```python
from build123d import *

# Parameters (mm, degrees)
CROQUIS1_R                      = 14
CROQUIS1_R_2                    = 4
SALIENTE_EXTRUIR1_DEPTH         = 18.9
CHAFL_N1_SIZE                   = 1
CORTAR_EXTRUIR1_REACH           = 44.671
REDONDEO1_R                     = 2
MATRIZC1_COUNT                  = 3
REDONDEO1_OF_MATRIZC1_R         = 2
CROQUIS3_R                      = 4
CORTAR_EXTRUIR2_DEPTH           = 29
TALADRO_ROSCADO_M3_5X0_61_D     = 2.9
TALADRO_ROSCADO_M3_5X0_61_DEPTH = 20
TALADRO_ROSCADO_M3_5X0_61_TIP   = 0.871247898
SALIENTE_EXTRUIR2_START         = -3
CROQUIS6_R                      = 18
CROQUIS6_R_2                    = 4
SALIENTE_EXTRUIR2_DEPTH         = 3
CHAFL_N2_SIZE                   = 0.5
REDONDEO2_R                     = 1


with BuildPart() as part:
    # Croquis1 → Saliente-Extruir1 (new, symmetric)
    with BuildSketch(Plane(origin=(0, 0, 0), x_dir=(0, 1, 0), z_dir=(0, 0, 1))):
        with Locations(Location((0, 0, 0), (0, 0, 270))):
            Circle(CROQUIS1_R)
        with Locations(Location((0, 0, 0), (0, 0, 270))):
            Circle(CROQUIS1_R_2, mode=Mode.SUBTRACT)
    extrude(amount=SALIENTE_EXTRUIR1_DEPTH, both=True)

    # Chaflán1
    chafl_n1_edges = [part.edges().sort_by_distance(p)[0] for p in [
        (-14, 0, 18.9),
    ]]
    chamfer(chafl_n1_edges, length=CHAFL_N1_SIZE)

    # Croquis2 → Cortar-Extruir1 (cut, up to next)
    with BuildSketch(Plane.XY.offset(18.9), mode=Mode.PRIVATE) as cortar_extruir1_sk1:
        with BuildLine():
            Line((4.022667121, 3.750753155), (4.08375287, 10.750486617))
            ThreePointArc((4.08375287, 10.750486617), (0, 11.5), (-4.08375287, 10.750486617))
            Line((-4.08375287, 10.750486617), (-4.022667121, 3.750753155))
            ThreePointArc((-4.022667121, 3.750753155), (0, 5.5), (4.022667121, 3.750753155))
        make_face()
    cortar_extruir1_tool1 = extrude(cortar_extruir1_sk1.sketch, amount=-CORTAR_EXTRUIR1_REACH, mode=Mode.PRIVATE) & part.part
    cortar_extruir1 = cortar_extruir1_tool1.solids().sort_by_distance((0, 8.096632, 18.9))[0]
    add(cortar_extruir1, mode=Mode.SUBTRACT)

    # Redondeo1
    redondeo1_edges = [part.edges().sort_by_distance(p)[0] for p in [
        (4.022667121, 3.750753155, 0),
        (-4.022667121, 3.750753155, 0),
        (-4.08375287, 10.750486617, 0),
        (4.08375287, 10.750486617, 0),
    ]]
    fillet(redondeo1_edges, radius=REDONDEO1_R)

    # MatrizC1: Cortar-Extruir1 ×3 about axis
    matrizc1_axis = Axis((0, 0, 0), (0, 0, 1))
    for i in range(1, MATRIZC1_COUNT):
        add(cortar_extruir1.rotate(matrizc1_axis, i * 360 / MATRIZC1_COUNT), mode=Mode.SUBTRACT)

    # Redondeo1 of MatrizC1
    redondeo1_of_matrizc1_edges = [part.edges().sort_by_distance(p)[0] for p in [
        (-5.259581076, 1.60835534, 0),
        (-1.236913955, -5.359108496, 0),
        (-7.268318079, -8.911877036, 0),
        (-11.352070948, -1.838609581, 0),
        (1.236913955, -5.359108496, 0),
        (5.259581076, 1.60835534, 0),
        (11.352070948, -1.838609581, 0),
        (7.268318079, -8.911877036, 0),
    ]]
    fillet(redondeo1_of_matrizc1_edges, radius=REDONDEO1_OF_MATRIZC1_R)

    # Croquis3 → Cortar-Extruir2 (cut)
    with BuildSketch(Plane(origin=(0, 0, 0), x_dir=(-1, 0, 0), z_dir=(0, 1, 0))):
        with Locations(Location((0, -0.4, 0), (0, 0, 90))):
            Circle(CROQUIS3_R)
    extrude(amount=-CORTAR_EXTRUIR2_DEPTH, mode=Mode.SUBTRACT)

    # Taladro roscado M3.5x0.61
    with Locations(Plane.XY.offset(18.9)):
        with Locations((0, 0), (-9.526279442, 5.5), (9.526279442, 5.5), (0, -11)):
            Hole(TALADRO_ROSCADO_M3_5X0_61_D / 2, depth=TALADRO_ROSCADO_M3_5X0_61_DEPTH)
            with Locations((0, 0, -(TALADRO_ROSCADO_M3_5X0_61_DEPTH + TALADRO_ROSCADO_M3_5X0_61_TIP / 2))):  # 118° drill point
                Cone(0, TALADRO_ROSCADO_M3_5X0_61_D / 2, TALADRO_ROSCADO_M3_5X0_61_TIP, mode=Mode.SUBTRACT)

    # Croquis6 → Saliente-Extruir2 (add)
    with BuildSketch(Plane(origin=(0, 0, -18.9), x_dir=(1, 0, 0), z_dir=(0, 0, -1)).offset(SALIENTE_EXTRUIR2_START)):
        with Locations(Location((0, 0, 0), (0, 0, 180))):
            Circle(CROQUIS6_R)
        Circle(CROQUIS6_R_2, mode=Mode.SUBTRACT)
        with BuildLine():
            Line((-10.049642775, 1.101731175), (-8.258409927, 0.08830039))
            ThreePointArc((-8.258409927, 0.08830039), (-6.485918981, -0.009361739), (-5.333946058, 1.341275307))
            ThreePointArc((-5.333946058, 1.341275307), (-4.763139721, 2.75), (-3.828551518, 3.948695135))
            ThreePointArc((-3.828551518, 3.948695135), (-3.234851986, 5.621651474), (-4.205675344, 7.107842597))
            Line((-4.205675344, 7.107842597), (-5.978948573, 8.152380354))
            ThreePointArc((-5.978948573, 8.152380354), (-7.288087529, 8.407385768), (-8.466451677, 7.782621409))
            ThreePointArc((-8.466451677, 7.782621409), (-9.959292144, 5.75), (-10.973173687, 3.440851528))
            ThreePointArc((-10.973173687, 3.440851528), (-10.92505342, 2.107976061), (-10.049642775, 1.101731175))
        make_face(mode=Mode.SUBTRACT)
        with BuildLine():
            Line((5.978948573, 8.152380354), (4.205675344, 7.107842597))
            ThreePointArc((4.205675344, 7.107842597), (3.234851986, 5.621651474), (3.828551518, 3.948695135))
            ThreePointArc((3.828551518, 3.948695135), (4.763139721, 2.75), (5.333946058, 1.341275307))
            ThreePointArc((5.333946058, 1.341275307), (6.485918981, -0.009361739), (8.258409927, 0.08830039))
            Line((8.258409927, 0.08830039), (10.049642775, 1.101731175))
            ThreePointArc((10.049642775, 1.101731175), (10.92505342, 2.107976061), (10.973173687, 3.440851528))
            ThreePointArc((10.973173687, 3.440851528), (9.959292144, 5.75), (8.466451677, 7.782621409))
            ThreePointArc((8.466451677, 7.782621409), (7.288087529, 8.407385768), (5.978948573, 8.152380354))
        make_face(mode=Mode.SUBTRACT)
        with BuildLine():
            Line((-4.052734583, -7.196142986), (-4.070694202, -9.254111529))
            ThreePointArc((-4.070694202, -9.254111529), (-3.63696589, -10.51536183), (-2.50672201, -11.223472937))
            ThreePointArc((-2.50672201, -11.223472937), (0, -11.5), (2.50672201, -11.223472937))
            ThreePointArc((2.50672201, -11.223472937), (3.63696589, -10.51536183), (4.070694202, -9.254111529))
            Line((4.070694202, -9.254111529), (4.052734583, -7.196142986))
            ThreePointArc((4.052734583, -7.196142986), (3.251066995, -5.612289735), (1.50539454, -5.289970442))
            ThreePointArc((1.50539454, -5.289970442), (0, -5.5), (-1.50539454, -5.289970442))
            ThreePointArc((-1.50539454, -5.289970442), (-3.251066995, -5.612289735), (-4.052734583, -7.196142986))
        make_face(mode=Mode.SUBTRACT)
    extrude(amount=SALIENTE_EXTRUIR2_DEPTH)

    # Chaflán2
    chafl_n2_edges = [part.edges().sort_by_distance(p)[0] for p in [
        (18, 0, -18.9),
        (18, 0, -15.9),
    ]]
    chamfer(chafl_n2_edges, length=CHAFL_N2_SIZE)

    # Redondeo2
    redondeo2_edges = [part.edges().sort_by_distance(p)[0] for p in [
        (-14, 0, -15.9),
    ]]
    fillet(redondeo2_edges, radius=REDONDEO2_R)


solid = part.part
```
Verification items for the finished model (mm, model axes). A direction names the side the tool comes from. Round coordinates to 2 decimals unless told otherwise and drop trailing zeros. Put each result on its own line as item: value. Start each with the question number.
(1) Depth check by flat-ended pin: pin 1 Ø1 at (x, z) = (4.5, 8.5) entering from -Y; pin 2 Ø3 at (y, z) = (-13, 13) entering from +X; pin 3 Ø12 at (x, z) = (-11.5, 9.5) entering from -Y; pin 4 Ø7 at (x, y) = (0, 0) entering from +Z. Enter the tip coordinate at first touch or a pass-through.
(2) Draft check along X on faces 1 (the face through (-13, 8, -15.9)), 2 (the face through (10.975, 5.564, 8.76)), 3 (the face through (13.267, 12.165, -17.386)). Enter one of: +X half, -X half, draft (parallel to the pull), parting line (faces both ways), or undercut.
(3) Tool access check on faces 4 (the face through (10.932, -2.126, -0.265)), 5 (the face through (-1.82, 13.88, 1.73)). Record the directions out of +Z, -Z, +X, -X, +Y, -Y that give a thin tool (end or side, any length) a straight path to the whole face; none if there is none.
(4) Material ranges on line 1 along Y through (x, z) = (0, 4); line 2 along X through (y, z) = (5, 12); line 3 along Z through (x, y) = (0, -7.5), recorded low to high.
(5) Section check A-A (x = 0). State how many separate pieces and enclosed holes the cut face has, then the cut area to 3 significant figures.
Completed:
1. pin 1: stops at y = -13.42
1. pin 2: stops at x = 7.98
1. pin 3: stops at y = -12.87
1. pin 4: passes through
2. face 1: draft
2. face 2: undercut
2. face 3: parting line
3. face 4: +Z, -Z
3. face 5: +Z
4. line 1: y = -14 to -12.45, -9.55 to -4, 4 to 5.5, 11.5 to 14
4. line 2: x = -13.08 to -10.89, -8.17 to 8.17, 10.89 to 13.08
4. line 3: z = -18.9 to -4.4, 3.6 to 18.9
5. separate pieces: 5
5. enclosed holes: 0
5. area: 428 mm2
